Geometry: final body of the model. Coordinates: model frame, mm. A direction names the side the tool comes from. Give positions to 0.01 mm unless a question says otherwise; leave off trailing zeros. Order: outer loops, then holes, each group sorted by start corner. A loop starts at its lowest first (then second) coordinate and runs counter-clockwise, first axis right, second up. Notation, with made-up numbers: (22.25, 14) -> (70.25, 14) arc R18 cw to (70.25, 23) -> close; hole circle Ø4 at (13.25, -38.75). An arc over 180 degrees is marked (long way). One line per item, written item: value. Start each with the question number.
```python
from build123d import *

# Parameters (mm, degrees)
F0_W     = 38.1
F0_H     = 12.7
F1_DEPTH = 2.54
F3_DEPTH = 38.1
F4_W     = 25.4
F4_H     = 2.921
F5_DEPTH = 12.7
F6_R     = 3.175
F7_DEPTH = 3


with BuildPart() as f1:
    # F0 (on Top) → F1 (new body)
    with BuildSketch(Plane.XY):
        with Locations((19.05, 6.35)):
            Rectangle(F0_W, F0_H)
    extrude(amount=F1_DEPTH)

    # F2 (on face) → F3 (join)
    with BuildSketch(Plane.YZ.offset(38.1)):
        Polygon((0, 2.54), (12.7, 2.54), (12.7, 7.62), (7.62, 7.62), align=None)
    extrude(amount=-F3_DEPTH)

    # F4 (on face) → F5 (cut)
    with BuildSketch(Plane.XZ):
        with Locations((19.05, 4.0005)):
            Rectangle(F4_W, F4_H)
    extrude(amount=-F5_DEPTH, mode=Mode.SUBTRACT)

    # F6 (on face) → F7 (join)
    with BuildSketch(Plane(origin=(0, 0, 0), x_dir=(1, 0, 0), z_dir=(0, 0, -1))):
        with Locations((11.43, -6.35)):
            Circle(F6_R)
        with Locations((26.67, -6.35)):
            Circle(F6_R)
    extrude(amount=F7_DEPTH)


solid = f1.part
```
1. Draft query along X for faces 1 (the cylindrical face through (29.6, 7.57, -1.48)), 2 (the flat face through (0, 8, 3)), 3 (the flat face through (19, 12.7, 2)). Return one class per face: pulls with the +X half, pulls with the -X half, needs draft (parallel to the pull), parting line crosses it, or undercut.
2. Access query for faces 4 (the flat face through (6.35, 8, 4)), 5 (the cylindrical face through (8.91, 8.28, -1.48)), 6 (the flat face through (11, 6, -3)). Directions: +Z, -Z, +X, -X, +Y, -Y. A direction counts if a zero-diameter tool reaches every point of the face in a straight line with its end or side. Return the directions, or none.
3. Pin query (flat end, axial travel): P1, Ø2.5, axis at x = 20.5, y = 10.5, coming from the -Z side; P2, Ø3, axis at x = 25.5, y = 2.5, coming from the +Z side. Return the tip coordinate at first contact, or that it passes through.
4. Cut plane D-D, the plane x = 26.67. Return loops of the section in (y, z) (1 decimal), then the cut area to 3 significant figures.
5. Cut plane B-B, the plane y = 5.75. Return loops of the section in (x, z), then the cut area to 3 significant figures.
6. Cut plane A-A, the plane x = 15.5. Return loops of the section in (y, z).
7. Cut plane C-C, the plane z = -1. Return loops of the section in (x, y) (3 decimals).
8. Material intervals for L1, parallel to Z at x = 19.5, y = 8.25; L2, parallel to Z at x = 13, y = 8.75; L3, parallel to X at y = 10, z = 3.25, sorted ascending. Write a range as [from, to].
Answers follow:
1. face 1: undercut
1. face 2: pulls with the -X half
1. face 3: needs draft
2. face 4: +Y, -Y
2. face 5: -Z
2. face 6: -Z, +X, -X, +Y, -Y
3. P1: stops at z = 0
3. P2: stops at z = 2.54
4. outline: (0, 0) -> (3.2, 0) -> (3.2, -3) -> (9.5, -3) -> (9.5, 0) -> (12.7, 0) -> (12.7, 2.5) -> (0, 2.5) -> close; (4.4, 5.5) -> (12.7, 5.5) -> (12.7, 7.6) -> (7.6, 7.6) -> close
4. area: 65.8 mm²
5. outline: (0, 0) -> (8.31, 0) -> (8.31, -3) -> (14.55, -3) -> (14.55, 0) -> (23.55, 0) -> (23.55, -3) -> (29.79, -3) -> (29.79, 0) -> (38.1, 0) -> (38.1, 6.37) -> (0, 6.37) -> close; hole (6.35, 2.54) -> (31.75, 2.54) -> (31.75, 5.46) -> (6.35, 5.46) -> close
5. area: 206 mm²
6. outline: (0, 0) -> (12.7, 0) -> (12.7, 2.54) -> (0, 2.54) -> close; (4.38, 5.46) -> (12.7, 5.46) -> (12.7, 7.62) -> (7.62, 7.62) -> close
7. outline: circle Ø6.35 at (11.43, 6.35); circle Ø6.35 at (26.67, 6.35)
8. L1: z = [0, 2.54], [5.46, 7.62]
8. L2: z = [-3, 2.54], [5.46, 7.62]
8. L3: x = [0, 6.35], [31.75, 38.1]
